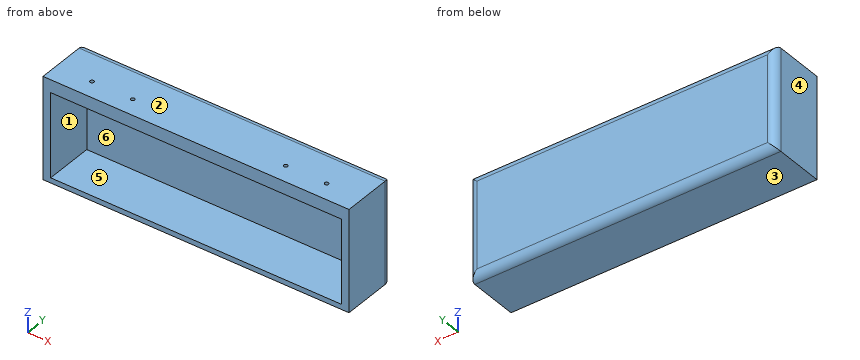
```python
from build123d import *

# Parameters (mm, degrees)
F0_W     = 120
F0_H     = 40
F1_DEPTH = 22
F2_W     = 114
F2_H     = 33
F3_DEPTH = 19
F4_R     = 3
F5_R     = 0.75
F6_DEPTH = 2


with BuildPart() as f1:
    # F0 (on Front) → F1 (new body)
    with BuildSketch(Plane.XZ):
        Rectangle(F0_W, F0_H)
    extrude(amount=F1_DEPTH)

    # F2 (on face) → F3 (cut)
    with BuildSketch(Plane.XZ.offset(22)):
        with Locations((0, -1.5)):
            Rectangle(F2_W, F2_H)
    extrude(amount=-F3_DEPTH, mode=Mode.SUBTRACT)

    # F4
    f4_edges = [f1.edges().sort_by_distance(p)[0] for p in [
        (0, 0, 20),
        (-60, 0, 0),
        (0, 0, -20),
        (60, 0, 0),
    ]]
    fillet(f4_edges, radius=F4_R)

    # F5 (on face) → F6 (cut)
    with BuildSketch(Plane.XY.offset(20)):
        with Locations((-46, -15)):
            Circle(F5_R)
        with Locations((-30, -15)):
            Circle(F5_R)
        with Locations((30, -15)):
            Circle(F5_R)
        with Locations((46, -15)):
            Circle(F5_R)
    extrude(amount=-F6_DEPTH, mode=Mode.SUBTRACT)


solid = f1.part
```
CAD build for the part. Positions are in the model's coordinates, mm. Face numbers are marked on the shaded views. A direction names the side the tool comes from. Coordinates: 2 decimals unless noted, no trailing zeros. Order: outer loops, then holes, each group sorted by start corner. A loop starts at its lowest first (then second) coordinate and runs counter-clockwise, first axis right, second up. Notation, with made-up numbers: (4, 27.5) -> (63, 27.5) arc R15 cw to (63, 53.5) -> close; hole circle Ø11 at (66.25, 35). An arc over 180 degrees is marked (long way). Use one line per item in the form item = value. Start each with the question number.
1) Band-saw the part on B-B on z = -0.5. Give the cut face in (x, y).
2) Band-saw the part on A-A on y = -10. Give the cut face in (x, z), then the cut area to 3 significant figures.
3) Drill centre lines: L1, parallel to Z at x = 12, y = -11; L2, parallel to X at y = -18, z = 5.5; L3, parallel to Y at x = -0.5, z = -3.5. Where is each one in solid material? Low to high. Write a range as [from, to].
4) Band-saw the part on C-C on x = -11. Give the cut face in (y, z).
5) Pull direction Z, two halves, no side cores. Call the marked faces 3, 4, 5 and 6: +Z half, -Z half, draft (parallel to the pull), parting line (faces both ways), or undercut.
6) Drop flat-ended pins along their axis: pin 1 (1.6 mm diameter, centred on x = 46, y = -15, fed in from +Z); pin 2 (1.2 mm diameter, centred on x = -30, y = -15, fed in from +Z); pin 3 (2 mm diameter, centred on x = -11.5, z = 9.5, fed in from -Y). Give the stop position or say it passes through.
7) Tool access for the marked faces 1 and 2: list every direction of +Z, -Z, +X, -X, +Y, -Y with a clear straight run to the whole face (end or side of a thin tool).
Entries:
q1.outline = (-60, -22) -> (-57, -22) -> (-57, -3) -> (57, -3) -> (57, -22) -> (60, -22) -> (60, -3) arc R3 ccw to (57, 0) -> (-57, 0) arc R3 ccw to (-60, -3) -> close
q2.outline = (-60, -20) -> (60, -20) -> (60, 20) -> (-60, 20) -> close; hole (-57, -18) -> (57, -18) -> (57, 15) -> (-57, 15) -> close
q2.area = 1,040 mm2
q3.L1 = [-20, -18], [15, 20]
q3.L2 = [-60, -57], [57, 60]
q3.L3 = [-3, 0]
q4.outline = (-22, -20) -> (-3, -20) arc R3 ccw to (0, -17) -> (0, 17) arc R3 ccw to (-3, 20) -> (-22, 20) -> (-22, 15) -> (-3, 15) -> (-3, -18) -> (-22, -18) -> close
q5.face_3 = -Z half
q5.face_4 = draft
q5.face_5 = undercut
q5.face_6 = undercut
q6.pin_1 = 20
q6.pin_2 = 18
q6.pin_3 = -3
q7.face_1 = -Y
q7.face_2 = +Z, +X, -X, +Y, -Y
